from build123d import *

# Parameters (mm, degrees)
SKETCH_1_W      = 6
SKETCH_1_H      = 1
EXTRUDE_1_DEPTH = 5
HOLE_WIZARD_0_D = 3.3


with BuildPart() as part:
    # 草图1 → 凸台-拉伸1 (new, symmetric)
    with BuildSketch(Plane.XY):
        Polygon((2.05, -0.813970588), (-2.05, -0.813970588), (-4.75, 1.886029412), (-4.75, 2.686029412), (4.75, 2.686029412), (4.75, 1.886029412), align=None)
        with Locations((0, 3.186029412)):
            Rectangle(SKETCH_1_W, SKETCH_1_H)
    extrude(amount=EXTRUDE_1_DEPTH, both=True)

    # Hole Wizard 0 (through all)
    with Locations(Plane(origin=(0, 3.686029412, 0), x_dir=(1, 0, 0), z_dir=(0, 1, 0))):
        with Locations((0, 0)):
            Hole(HOLE_WIZARD_0_D / 2)


solid = part.part
For this review, take the finished solid that the model builds, in its own axes (mm). A direction names the side the tool comes from. Give positions to 0.01 mm unless a question says otherwise; leave off trailing zeros. Loops run counter-clockwise (first coordinate to the right, second up) from the corner with the lowest first, then second, coordinate; pieces in that order, holes last. Notation, with made-up numbers: M -3.75,88 L 40.25,88 A29 ccw 40.25,117 Z; hole C -32.75,-8 d11. An arc over 180 degrees is marked long. Put each result on its own line as item: value. Start each with the question number.
(1) Machinability: for faces 4 (the flat face through (3, 3, 0)), 5 (the flat face through (-3.381, 0.517, 0.07)), 6 (the flat face through (-3, 3, 0)), which of the approach directions +Z, -Z, +X, -X, +Y, -Y give a long, thin tool a straight path to every point of the face, cutting with its end or side? Answer none if there is none.
(2) Add section B-B, the plane x = 0. Write out the cut boundary in (y, z), then the cut area to 4 significant figures.
(3) For pin 1 (2.5 mm diameter, centred on x = 0, z = 0, fed in from +Y); pin 2 (0.9 mm diameter, centred on x = -3.5, z = 0.5, fed in from +Y); pin 3 (0.8 mm diameter, centred on y = 3.5, z = -1, fed in from -X); pin 4 (1.5 mm diameter, centred on x = -3.5, z = 2.5, fed in from -Y), all flat-tipped, find the tip position at first contact; note any pin that passes through.
(4) Add section C-C, the plane y = 2.4. Write out the cut boundary in (x, z).
(5) Add section A-A, the plane z = 0. Write out the cut boundary in (x, y), then the cut area to 3 significant figures.
(6) Add section D-D, the plane z = -3. Write out the cut boundary in (x, y).
(7) Wall thickness on L1, parallel to Z at x = 0, y = 1.75; L2, parallel to X at y = 1.8, z = 1; L3, parallel to X at y = 3.05, z = 1: over which ranges is each line inside the solid? List them lowest first.
(8) The part is to be moulded in two halves that separate along Z. For faces 1 (the flat face through (0, 1, -5)), 2 (the flat face through (-4, 2.686, 0)), 3 (the cylindrical face through (1.216, 1.405, -1.115)), say which applies: +Z half, -Z half, draft (parallel to the pull), parting line (faces both ways), or undercut.
Result:
1. face 4: +Z, -Z, +X, +Y
1. face 5: +Z, -Z, -X, -Y
1. face 6: +Z, -Z, -X, +Y
2. outline: M -0.81,-5 L 3.69,-5 L 3.69,-1.65 L -0.81,-1.65 Z; M -0.81,1.65 L 3.69,1.65 L 3.69,5 L -0.81,5 Z
2. area: 30.15 mm^2
3. pin 1: passes through
3. pin 2: stops at y = 2.69
3. pin 3: stops at x = -3
3. pin 4: stops at y = -0.11
4. outline: M -4.75,-5 L 4.75,-5 L 4.75,5 L -4.75,5 Z; hole C 0,0 d3.3
5. outline: M -4.75,1.89 L -2.05,-0.81 L -1.65,-0.81 L -1.65,3.69 L -3,3.69 L -3,2.69 L -4.75,2.69 Z; M 1.65,-0.81 L 2.05,-0.81 L 4.75,1.89 L 4.75,2.69 L 3,2.69 L 3,3.69 L 1.65,3.69 Z
5. area: 17.1 mm^2
6. outline: M -4.75,1.89 L -2.05,-0.81 L 2.05,-0.81 L 4.75,1.89 L 4.75,2.69 L 3,2.69 L 3,3.69 L -3,3.69 L -3,2.69 L -4.75,2.69 Z
7. L1: z = -5 to -1.65, 1.65 to 5
7. L2: x = -4.66 to -1.31, 1.31 to 4.66
7. L3: x = -3 to -1.31, 1.31 to 3
8. face 1: -Z half
8. face 2: draft
8. face 3: undercut
